Answer from the drawing. Dimensions are ordinates in mm from the lowest x, y and z of the part. A direction names the side the tool comes from. Round coordinates to 2 decimals unless told otherwise and drop trailing zeros. Write each loop counter-clockwise with the first axis right and the second up, starting at its lowest first coordinate (ties: lowest second). Pieces come first, ordered by that corner, then holes. Notation, with made-up numbers: (71, 20) - (113, 20) arc R27 cw to (113, 44) - close; hole circle Ø3 at (-29.75, 25). An arc over 180 degrees is marked (long way). Answer as CSV lines item,"result". Start each with the question number.
1) For a pull along X with two mould halves and no side action, classify the marked faces 1, 2 and 3 as +X half, -X half, draft (parallel to the pull), parting line (faces both ways), or undercut.
2) Find section D-D on y = 42. Determine the outline of the cut face in (x, z).
3) Consider line 1 along X through (y, z) = (34.5, 6.25); line 2 along Y through (x, z) = (35, 4.25); line 3 along X through (y, z) = (41, 3.5). Determine where each line is inside the solid, lowest interval first.
4) Find section A-A on x = 35. Determine the outline of the cut face in (y, z).
5) Find section C-C on z = 4.5. Determine the outline of the cut face in (x, y), then the cut area to 3 significant figures.
6) Each of these flat-tipped pins is pushed along its axis until it touches: pin 1 (8.5 mm diameter, centred on x = 15, y = 35.5, fed in from +Z); pin 2 (3 mm diameter, centred on x = 31.5, z = 3.5, fed in from -Y); pin 3 (2 mm diameter, centred on x = 45, z = 1, fed in from -Y). Where does it stop, or does it pass through?
7) Find section B-B on y = 35. Determine the outline of the cut face in (x, z) (3 decimals).
8) Which of the six approach directions +Z, -Z, +X, -X, +Y, -Y give full straight-line access (tool end or side, diameter ignored) to the marked faces 4 and 5?
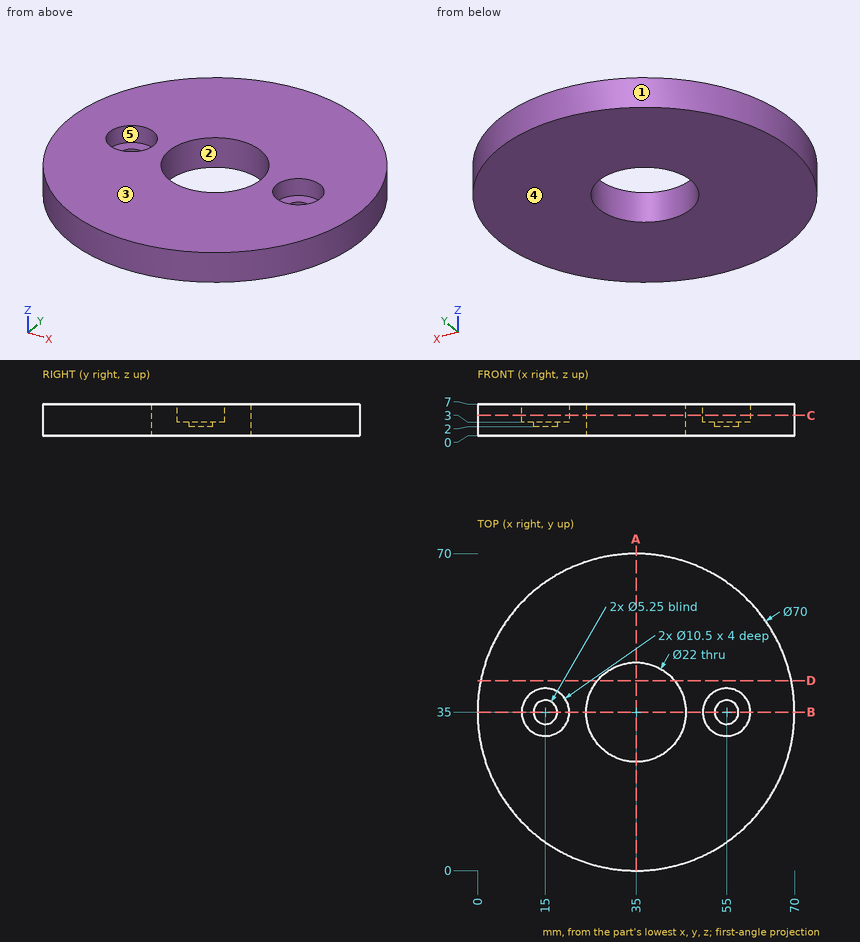
Check values:
1,face 1,"parting line"
1,face 2,"undercut"
1,face 3,"draft"
2,outline,"(0.71, 0) - (26.51, 0) - (26.51, 7) - (0.71, 7) - close; (43.49, 0) - (69.29, 0) - (69.29, 7) - (43.49, 7) - close"
3,line 1,"x = 0 to 9.77, 20.23 to 24.01, 45.99 to 49.77, 60.23 to 70"
3,line 2,"y = 0 to 24, 46 to 70"
3,line 3,"x = 0.52 to 25.78, 44.22 to 69.48"
4,outline,"(0, 0) - (24, 0) - (24, 7) - (0, 7) - close; (46, 0) - (70, 0) - (70, 7) - (46, 7) - close"
5,outline,"circle Ø70 at (35, 35); hole circle Ø10.5 at (15, 35); hole circle Ø22 at (35, 35); hole circle Ø10.5 at (55, 35)"
5,area,"3,300 mm^2"
6,pin 1,"stops at z = 3"
6,pin 2,"stops at y = 0.06"
6,pin 3,"stops at y = 1.18"
7,outline,"(0, 0) - (24, 0) - (24, 7) - (20.25, 7) - (20.25, 3) - (17.625, 3) - (17.625, 2) - (12.375, 2) - (12.375, 3) - (9.75, 3) - (9.75, 7) - (0, 7) - close; (46, 0) - (70, 0) - (70, 7) - (60.25, 7) - (60.25, 3) - (57.625, 3) - (57.625, 2) - (52.375, 2) - (52.375, 3) - (49.75, 3) - (49.75, 7) - (46, 7) - close"
8,face 4,"-Z, +X, -X, +Y, -Y"
8,face 5,"+Z"
